```python
from build123d import *

# Parameters (mm, degrees)
F2_DEPTH = 29.5
F3_DEPTH = 30
F5_DEPTH = 45.85
F6_W     = 9
F6_H     = 4
F7_DEPTH = 12.5
F8_W     = 4
F8_H     = 4
F9_DEPTH = 12.5


with BuildPart() as f2:
    # F0 (on Right) → F2 (new body, symmetric)
    with BuildSketch(Plane.YZ):
        Polygon((11, 0), (5.5, 9.526279), (-5.5, 9.526279), (-11, 0), (-5.5, -9.526279), (5.5, -9.526279), align=None)
    extrude(amount=F2_DEPTH, both=True)

    # F1 (on Right) → F3 (cut, symmetric)
    with BuildSketch(Plane.YZ):
        Polygon((-5.03812, 8.726279), (-10.07624, 0), (-5.03812, -8.726279), (5.03812, -8.726279), (10.07624, 0), (5.03812, 8.726279), align=None)
    extrude(amount=F3_DEPTH, both=True, mode=Mode.SUBTRACT)

    # F4 (on face) → F5 (cut, symmetric)
    with BuildSketch(Plane.YZ):
        Polygon((-12.379561, 14.501398), (-12.379561, 2.501398), (-9.555817, 2.501398), (-5.5, 9.526279), (5.5, 9.526279), (9.555817, 2.501398), (12.266592, 2.501398), (12.266592, 14.501398), align=None)
        Polygon((-5.5, 9.526279), (-9.555817, 2.501398), (9.555817, 2.501398), (5.5, 9.526279), align=None)
    extrude(amount=F5_DEPTH, both=True, mode=Mode.SUBTRACT)

    # F6 (on Front) → F7 (cut, symmetric)
    with BuildSketch(Plane.XZ):
        with Locations((11, -3.526279)):
            Rectangle(F6_W, F6_H)
        with Locations((-11, -3.526279)):
            Rectangle(F6_W, F6_H)
    extrude(amount=F7_DEPTH, both=True, mode=Mode.SUBTRACT)

    # F8 (on Front) → F9 (cut, symmetric)
    with BuildSketch(Plane.XZ):
        with Locations((-27.774018, 0.550773)):
            Rectangle(F8_W, F8_H)
        with Locations((27.774018, 0.550773)):
            Rectangle(F8_W, F8_H)
    extrude(amount=F9_DEPTH, both=True, mode=Mode.SUBTRACT)


solid = f2.part
```
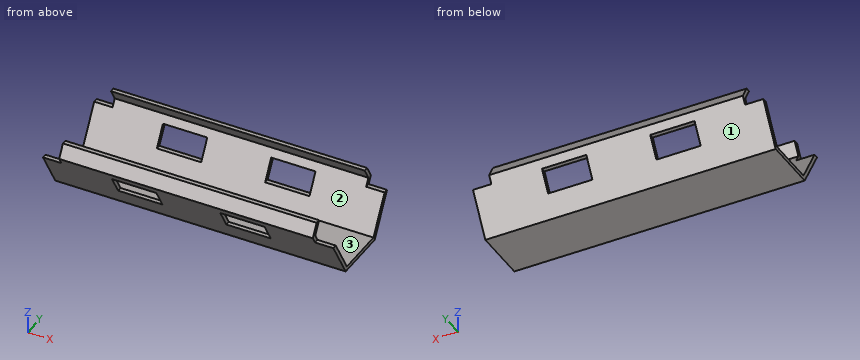
Could you check a few things on this model? Use its own coordinates, in mm. Face numbers are marked on the shaded views. Give positions to 0.01 mm unless a question says otherwise; leave off trailing zeros. Loops run counter-clockwise (first coordinate to the right, second up) from the corner with the lowest first, then second, coordinate; pieces in that order, holes last. Notation, with made-up numbers: (7.25, 20.5) - (38.25, 20.5) arc R16 cw to (38.25, 50.5) - close; hole circle Ø11 at (59, 16). An arc over 180 degrees is marked (long way). Use one line per item in the form item = value.
1. I want a section at A-A (x = -9.5). Please give me the cut outline in (y, z), and give its area (3 significant figures).
Response values:
outline = (-11, 0) - (-10.12, -1.53) - (-9.2, -1.53) - (-10.08, 0) - (-8.63, 2.5) - (-9.56, 2.5) - close; (-7.81, -5.53) - (-5.5, -9.53) - (5.5, -9.53) - (7.81, -5.53) - (6.89, -5.53) - (5.04, -8.73) - (-5.04, -8.73) - (-6.89, -5.53) - close; (8.63, 2.5) - (10.08, 0) - (9.2, -1.53) - (10.12, -1.53) - (11, 0) - (9.56, 2.5) - close
area = 22.5 mm²
2. Thinking about a two-plate mould opening in Z: for the marked faces 1, 2 and 3, which applies, released by +Z, released by -Z, zero draft, split by the parting line, or undercut?
Response values:
face_1 = released by -Z
face_2 = undercut
face_3 = released by +Z
3. I'm going to push flat-ended pins straight in: pin 1 Ø1.5 at (x, y) = (-11, 1.5) entering from +Z; pin 2 Ø1.2 at (y, z) = (-9.5, 1) entering from -X; pin 3 Ø2.5 at (y, z) = (10.5, 0) entering from +X. Where does each tip first touch, or does it pass through?
Response values:
pin_1 = -8.73
pin_2 = -25.77
pin_3 = 25.77
4. I need wall thicknesses on probe 1 along Y at (x, z) = (13, -8.5); probe 2 along Z at (x, y) = (5, -2.25); probe 3 along Y at (x, z) = (15.5, -6.5). Which ranges of each line are inside material? Lowest first, please.
Response values:
probe_1 = -6.09 to -5.17, 5.17 to 6.09
probe_2 = -9.53 to -8.73
probe_3 = -7.25 to -6.32, 6.32 to 7.25
5. I want a section at C-C (z = -2.25). Please give me the cut outline in (x, y), and give its area (3 significant figures).
Response values:
outline = (-29.5, -9.7) - (-15.5, -9.7) - (-15.5, -8.78) - (-29.5, -8.78) - close; (-29.5, 8.78) - (-15.5, 8.78) - (-15.5, 9.7) - (-29.5, 9.7) - close; (-6.5, -9.7) - (6.5, -9.7) - (6.5, -8.78) - (-6.5, -8.78) - close; (-6.5, 8.78) - (6.5, 8.78) - (6.5, 9.7) - (-6.5, 9.7) - close; (15.5, -9.7) - (29.5, -9.7) - (29.5, -8.78) - (15.5, -8.78) - close; (15.5, 8.78) - (29.5, 8.78) - (29.5, 9.7) - (15.5, 9.7) - close
area = 75.7 mm²
6. I want a section at B-B (z = -8). Please give me the cut outline in (x, y), and give its area (3 significant figures).
Response values:
outline = (-29.5, -6.38) - (29.5, -6.38) - (29.5, -5.46) - (-29.5, -5.46) - close; (-29.5, 5.46) - (29.5, 5.46) - (29.5, 6.38) - (-29.5, 6.38) - close
area = 109 mm²
7. I want a section at D-D (x = -24). Please give me the cut outline in (y, z).
Response values:
outline = (-11, 0) - (-5.5, -9.53) - (5.5, -9.53) - (11, 0) - (9.56, 2.5) - (8.63, 2.5) - (10.08, 0) - (5.04, -8.73) - (-5.04, -8.73) - (-10.08, 0) - (-8.63, 2.5) - (-9.56, 2.5) - close
